Work out the finished part from the listing and answer in its coordinate system (mm). A direction names the side the tool comes from. Round coordinates to 2 decimals unless told otherwise and drop trailing zeros. Order: outer loops, then holes, each group sorted by start corner. A loop starts at its lowest first (then second) coordinate and runs counter-clockwise, first axis right, second up. Notation, with made-up numbers: (-2.5, -35) - (16.5, -35) arc R12 cw to (16.5, -13) - close; hole circle Ø5 at (-37.5, 60.5). An arc over 180 degrees is marked (long way). Put each result on its own line as item: value.
Autodesk Inventor part; units mm, degrees
ref_plane "D_XY" through (0, 0, 0) normal (0, 1, 0) x (1, 0, 0)
ref_plane "D_YZ" through (0, 0, 0) normal (1, 0, 0) x (0, 0, -1)
ref_plane "D_ZX" through (0, 0, 0) normal (0, 0, -1) x (0, 1, 0)
sketch "Sketch_2" plane through (0, 0, 0) normal (0, 0, 1) x (1, 0, 0)
  line L0 (-12.0015, 8.6106) -> (-10.9982, 8.6106)
  line L1 (-10.9982, 8.6106) -> (-10.9982, 3.81)
  line L2 (-10.9982, 3.81) -> (-10.8712, 3.81)
  line L3 (-10.8712, 3.81) -> (-10.8712, 1.27)
  line L4 (-10.8712, 1.27) -> (-10.9982, 1.27)
  line L5 (-10.9982, 1.27) -> (-10.9982, 0)
  line L6 (-10.9982, 0) -> (10.9982, 0)
  line L7 (10.9982, 0) -> (10.9982, 1.27)
  line L8 (10.9982, 1.27) -> (10.8712, 1.27)
  line L9 (10.8712, 1.27) -> (10.8712, 3.81)
  line L10 (10.8712, 3.81) -> (10.9982, 3.81)
  line L11 (10.9982, 3.81) -> (10.9982, 8.6106)
  line L12 (10.9982, 8.6106) -> (12.0015, 8.6106)
  line L13 (12.0015, 8.6106) -> (12.0015, 8.8646)
  line L14 (12.0015, 8.8646) -> (10.3691, 10.0076)
  line L15 (10.3691, 10.0076) -> (-10.3691, 10.0076)
  line L16 (-10.3691, 10.0076) -> (-12.0015, 8.8646)
  line L17 (-12.0015, 8.8646) -> (-12.0015, 8.6106)
extrude "Extrusion1" add sketch "Sketch_2" along normal mid plane 24.003
sketch "Sketch_1" plane through (0, 0, 0) normal (1, 0, 0) x (0, 1, 0)
  line L0 (12.7, 12.7) -> (-2.54, 12.7)
  line L1 (-2.54, 12.7) -> (-2.54, -12.7)
  line L2 (-2.54, -12.7) -> (12.7, -12.7)
  line L3 (12.7, -12.7) -> (12.7, 12.7)
  line L4 (8.6106, 8.9027) -> (8.6106, 7.7724)
  line L5 (8.6106, 7.7724) -> (1.27, 7.7724)
  line L6 (1.27, 7.7724) -> (1.27, 7.8994)
  line L7 (1.27, 7.8994) -> (0, 7.8994)
  line L8 (0, 7.8994) -> (0, -7.8994)
  line L9 (0, -7.8994) -> (1.27, -7.8994)
  line L10 (1.27, -7.8994) -> (1.27, -7.7724)
  line L11 (1.27, -7.7724) -> (8.6106, -7.7724)
  line L12 (8.6106, -7.7724) -> (8.6106, -8.9027)
  line L13 (8.6106, -8.9027) -> (8.8646, -8.9027)
  line L14 (8.8646, -8.9027) -> (10.0076, -7.2703)
  line L15 (10.0076, -7.2703) -> (10.0076, 7.2703)
  line L16 (10.0076, 7.2703) -> (8.8646, 8.9027)
  line L17 (8.8646, 8.9027) -> (8.6106, 8.9027)
extrude "Extrusion2" cut sketch "Sketch_1" along normal mid plane 25.4
sketch "Sketch_3" plane through (0, 10.0076, 0) normal (0, 1, 0) x (1, 0, 0)
  line L0 (-8.4963, 5.4864) -> (-8.4963, -5.4864)
  arc A0 (-8.4963, -5.4864) -> (-7.9883, -5.9944) centre (-7.9883, -5.4864) ccw
  line L1 (-7.9883, -5.9944) -> (7.9883, -5.9944)
  arc A1 (7.9883, -5.9944) -> (8.4963, -5.4864) centre (7.9883, -5.4864) ccw
  line L2 (8.4963, -5.4864) -> (8.4963, 5.4864)
  arc A2 (8.4963, 5.4864) -> (7.9883, 5.9944) centre (7.9883, 5.4864) ccw
  line L3 (7.9883, 5.9944) -> (-7.9883, 5.9944)
  arc A3 (-7.9883, 5.9944) -> (-8.4963, 5.4864) centre (-7.9883, 5.4864) ccw
sketch "Sketch_4" plane through (0, 0, 0) normal (0, 1, 0) x (-1, 0, 0)
  line L0 (10.9982, -6.6294) -> (10.9982, 6.6294)
  line L1 (10.9982, 6.6294) -> (9.7282, 6.6294)
  line L2 (9.7282, 6.6294) -> (9.7282, 7.8994)
  line L3 (9.7282, 7.8994) -> (-9.7282, 7.8994)
  line L4 (-9.7282, 7.8994) -> (-9.7282, 6.6294)
  line L5 (-9.7282, 6.6294) -> (-10.9982, 6.6294)
  line L6 (-10.9982, 6.6294) -> (-10.9982, 1.27)
  line L7 (-10.9982, 1.27) -> (-9.7282, 1.27)
  line L8 (-9.7282, 1.27) -> (-9.7282, -1.27)
  line L9 (-9.7282, -1.27) -> (-10.9982, -1.27)
  line L10 (-10.9982, -1.27) -> (-10.9982, -6.6294)
  line L11 (-10.9982, -6.6294) -> (-9.7282, -6.6294)
  line L12 (-9.7282, -6.6294) -> (-9.7282, -7.8994)
  line L13 (-9.7282, -7.8994) -> (9.7282, -7.8994)
  line L14 (9.7282, -7.8994) -> (9.7282, -6.6294)
  line L15 (9.7282, -6.6294) -> (10.9982, -6.6294)
extrude "Extrusion3" cut sketch "Sketch_4" along normal blind 0.2032
sketch "Sketch_6" plane through (0, 0, 0) normal (0, 1, 0) x (-1, 0, 0)
  line L0 (9.7282, 7.1374) -> (1.27, 7.1374)
  line L1 (1.27, 7.1374) -> (1.27, 7.3914)
  line L2 (1.27, 7.3914) -> (-1.27, 7.3914)
  line L3 (-1.27, 7.3914) -> (-1.27, 7.1374)
  line L4 (-1.27, 7.1374) -> (-9.7282, 7.1374)
  line L5 (-9.7282, 7.1374) -> (-9.7282, -7.1374)
  line L6 (-9.7282, -7.1374) -> (9.7282, -7.1374)
  line L7 (9.7282, -7.1374) -> (9.7282, 7.1374)
extrude "Extrusion4" cut sketch "Sketch_6" along normal blind 0.4064
sketch "Sketch_9" plane through (0, 0, 0) normal (1, 0, 0) x (0, 1, 0)
  line L0 (1.27, 2.54) -> (1.27, -2.54)
  line L1 (1.27, -2.54) -> (3.81, -2.54)
  line L2 (3.81, -2.54) -> (3.81, 2.54)
  line L3 (3.81, 2.54) -> (1.27, 2.54)
extrude "Extrusion5" add sketch "Sketch_9" along normal mid plane 21.9964
sketch "Sketch_8" plane through (0, 2.54, 0) normal (0, 1, 0) x (1, 0, 0)
  line L0 (-10.9982, -4.5974) -> (-10.7442, -5.3594)
  line L1 (-10.7442, -5.3594) -> (-10.7442, -6.6294)
  line L2 (-10.7442, -6.6294) -> (10.7442, -6.6294)
  line L3 (10.7442, -6.6294) -> (10.7442, -5.3594)
  line L4 (10.7442, -5.3594) -> (10.9982, -4.5974)
  line L5 (10.9982, -4.5974) -> (10.9982, -4.0894)
  line L6 (10.9982, -4.0894) -> (10.7442, -4.0894)
  line L7 (10.7442, -4.0894) -> (10.7442, 4.0894)
  line L8 (10.7442, 4.0894) -> (10.9982, 4.0894)
  line L9 (10.9982, 4.0894) -> (10.9982, 4.5974)
  line L10 (10.9982, 4.5974) -> (10.7442, 5.3594)
  line L11 (10.7442, 5.3594) -> (10.7442, 6.6294)
  line L12 (10.7442, 6.6294) -> (-10.7442, 6.6294)
  line L13 (-10.7442, 6.6294) -> (-10.7442, 5.3594)
  line L14 (-10.7442, 5.3594) -> (-10.9982, 4.5974)
  line L15 (-10.9982, 4.5974) -> (-10.9982, 4.0894)
  line L16 (-10.9982, 4.0894) -> (-10.7442, 4.0894)
  line L17 (-10.7442, 4.0894) -> (-10.7442, -4.0894)
  line L18 (-10.7442, -4.0894) -> (-10.9982, -4.0894)
  line L19 (-10.9982, -4.0894) -> (-10.9982, -4.5974)
extrude "Extrusion6" add sketch "Sketch_8" along normal mid plane 0.508
sketch "Sketch_19" plane through (0, 0, 0) normal (0, 0, 1) x (1, 0, 0)
  line L0 (-8.4582, 3.048) -> (8.4582, 3.048)
  line L1 (8.4582, 3.048) -> (8.4582, 8.6868)
  line L2 (8.4582, 8.6868) -> (-8.4582, 8.6868)
  line L3 (-8.4582, 8.6868) -> (-8.4582, 3.048)
extrude "Extrusion7" add sketch "Sketch_19" along normal mid plane 15.7988
extrude "Extrusion8" cut sketch "Sketch_3" against normal blind 5.08
ref_plane "D_XY" through (0, 0, 0) normal (0, 1, 0) x (1, 0, 0)
ref_plane "D_YZ" through (0, 0, 0) normal (1, 0, 0) x (0, 0, -1)
ref_plane "D_ZX" through (0, 0, 0) normal (0, 0, -1) x (0, 1, 0)
ref_plane "LENS_XY" through (0, 10.0076, 0) normal (0, -1, 0) x (1, 0, 0)
ref_plane "LENS_YZ" through (0, 10.0076, 0) normal (1, 0, 0) x (0, 0, 1)
ref_plane "LENS_ZX" through (0, 10.0076, 0) normal (0, 0, 1) x (0, -1, 0)
ref_plane "P_1_XY" through (7.62, 0.4064, 5.08) normal (0, 1, 0) x (1, 0, 0)
ref_plane "P_1_YZ" through (7.62, 0.4064, 5.08) normal (1, 0, 0) x (0, 0, -1)
ref_plane "P_1_ZX" through (7.62, 0.4064, 5.08) normal (0, 0, -1) x (0, 1, 0)
ref_plane "P_2_XY" through (7.62, 0.4064, 0) normal (0, 1, 0) x (1, 0, 0)
ref_plane "P_2_YZ" through (7.62, 0.4064, 0) normal (1, 0, 0) x (0, 0, -1)
ref_plane "P_2_ZX" through (7.62, 0.4064, 0) normal (0, 0, -1) x (0, 1, 0)
ref_plane "P_3_XY" through (7.62, 0.4064, -5.08) normal (0, 1, 0) x (1, 0, 0)
ref_plane "P_3_YZ" through (7.62, 0.4064, -5.08) normal (1, 0, 0) x (0, 0, -1)
ref_plane "P_3_ZX" through (7.62, 0.4064, -5.08) normal (0, 0, -1) x (0, 1, 0)
ref_plane "P_4_XY" through (0, 0.4064, 2.54) normal (0, 1, 0) x (1, 0, 0)
ref_plane "P_4_YZ" through (0, 0.4064, 2.54) normal (1, 0, 0) x (0, 0, -1)
ref_plane "P_4_ZX" through (0, 0.4064, 2.54) normal (0, 0, -1) x (0, 1, 0)
ref_plane "P_5_XY" through (0, 0.4064, -2.54) normal (0, 1, 0) x (1, 0, 0)
ref_plane "P_5_YZ" through (0, 0.4064, -2.54) normal (1, 0, 0) x (0, 0, -1)
ref_plane "P_5_ZX" through (0, 0.4064, -2.54) normal (0, 0, -1) x (0, 1, 0)
ref_plane "body_to_metal_1_XY" through (0, 0, 0) normal (0, -1, 0) x (1, 0, 0)
ref_plane "body_to_metal_1_YZ" through (0, 0, 0) normal (1, 0, 0) x (0, 0, 1)
ref_plane "body_to_metal_1_ZX" through (0, 0, 0) normal (0, 0, 1) x (0, -1, 0)
ref_plane "body_to_metal_2_XY" through (0, 0, 0) normal (0, -1, 0) x (1, 0, 0)
ref_plane "body_to_metal_2_YZ" through (0, 0, 0) normal (1, 0, 0) x (0, 0, 1)
ref_plane "body_to_metal_2_ZX" through (0, 0, 0) normal (0, 0, 1) x (0, -1, 0)
properties part number "UB16NKG015F-NR"
1) For a pull along Z with two mould halves and no side action, classify faces 6 (the flat face through (10, 0, 0)), 7 (the flat face through (0, 8, -5.994)), 8 (the flat face through (8.496, 8, 0)), 9 (the flat face through (-0.17, 9.44, 8.08)) as pulls with the +Z half, pulls with the -Z half, needs draft (parallel to the pull), parting line crosses it, or undercut.
Findings below:
face 6: needs draft
face 7: undercut
face 8: undercut
face 9: pulls with the +Z half
2) A cutting plane is placed at C-C on x = -1. Write down the section's boundary in (y, z).
Findings below:
outline: (0.2, -7.9) - (1.27, -7.9) - (1.27, -7.77) - (3.05, -7.77) - (3.05, -7.9) - (8.61, -7.9) - (8.61, -8.9) - (8.86, -8.9) - (10.01, -7.27) - (10.01, -5.99) - (4.93, -5.99) - (4.93, 5.99) - (10.01, 5.99) - (10.01, 7.27) - (8.86, 8.9) - (8.61, 8.9) - (8.61, 7.9) - (3.05, 7.9) - (3.05, 7.77) - (1.27, 7.77) - (1.27, 7.9) - (0.2, 7.9) - (0.2, 7.39) - (0.41, 7.39) - (0.41, -7.14) - (0.2, -7.14) - close
3) Given pin 1 Ø1 at (y, z) = (1.5, 6) entering from -X; pin 2 Ø4 at (x, y) = (2, 4.5) entering from +Z; pin 3 Ø1 at (x, z) = (0.5, -1.5) entering from -Y, each flat-ended and moving along its own axis, determine where each tip first touches the part or whether it passes through.
Findings below:
pin 1: stops at x = -11
pin 2: stops at z = 7.9
pin 3: stops at y = 0.41
4) A cutting plane is placed at A-A on z = 0.25. Write down the section's boundary in (x, y), then the cut area to 3 significant figures.
Findings below:
outline: (-12, 8.61) - (-11, 8.61) - (-11, 0.2) - (-9.73, 0.2) - (-9.73, 0.41) - (9.73, 0.41) - (9.73, 0) - (11, 0) - (11, 8.61) - (12, 8.61) - (12, 8.86) - (10.37, 10.01) - (8.5, 10.01) - (8.5, 4.93) - (-8.5, 4.93) - (-8.5, 10.01) - (-10.37, 10.01) - (-12, 8.86) - close
area: 127 mm2
5) A cutting plane is placed at D-D on z = 3. Write down the section's boundary in (x, y), then the cut area to 3 significant figures.
Findings below:
outline: (-12, 8.61) - (-11, 8.61) - (-11, 3.81) - (-10.87, 3.81) - (-10.87, 1.27) - (-11, 1.27) - (-11, 0.2) - (-9.73, 0.2) - (-9.73, 0.41) - (9.73, 0.41) - (9.73, 0.2) - (11, 0.2) - (11, 1.27) - (10.87, 1.27) - (10.87, 3.81) - (11, 3.81) - (11, 8.61) - (12, 8.61) - (12, 8.86) - (10.37, 10.01) - (8.5, 10.01) - (8.5, 4.93) - (-8.5, 4.93) - (-8.5, 10.01) - (-10.37, 10.01) - (-12, 8.86) - close
area: 126 mm2
6) A cutting plane is placed at B-B on y = 7.25. Write down the section's boundary in (x, z), then the cut area to 3 significant figures.
Findings below:
outline: (-11, -7.77) - (-8.46, -7.77) - (-8.46, -7.9) - (8.46, -7.9) - (8.46, -7.77) - (11, -7.77) - (11, 7.77) - (8.46, 7.77) - (8.46, 7.9) - (-8.46, 7.9) - (-8.46, 7.77) - (-11, 7.77) - close; hole (-8.5, -5.49) arc R0.51 ccw to (-7.99, -5.99) - (7.99, -5.99) arc R0.51 ccw to (8.5, -5.49) - (8.5, 5.49) arc R0.51 ccw to (7.99, 5.99) - (-7.99, 5.99) arc R0.51 ccw to (-8.5, 5.49) - close
area: 143 mm2
7) Straight lines are drawn through the part: L1, parallel to X at y = 6, z = -3.5; L2, parallel to Z at x = 4.5, y = 5.5; L3, parallel to Z at x = 10, y = 2.5. For each, find the intervals that lie inside material, in ascending order. Write a range as from..to.
Findings below:
L1: x = -11..-8.5, 8.5..11
L2: z = -7.9..-5.99, 5.99..7.9
L3: z = -7.77..7.77
8) For faces 1 (the flat face through (10.998, 5, 0)), 2 (the flat face through (0, 4.928, 0)), 3 (the flat face through (0, 6, -7.899)), 4 (the flat face through (0, 6, 7.899)), 5 (the flat face through (-11.174, 9.444, -0.125)), determine the directions among +Z, -Z, +X, -X, +Y, -Y from which every point of the face is accessible in a straight line to the end or side of a thin tool.
Findings below:
face 1: +Z, -Z, +X, -Y
face 2: +Y
face 3: -Z, +X, -X, -Y
face 4: +Z, +X, -X, -Y
face 5: +Z, -Z, -X, +Y
